Part model, mm, in its own coordinate system. A direction names the side the tool comes from. Round coordinates to 2 decimals unless told otherwise and drop trailing zeros. Loops run counter-clockwise (first coordinate to the right, second up) from the corner with the lowest first, then second, coordinate; pieces in that order, holes last. Notation, with made-up numbers: (-21, -9) - (-14, -9) arc R25 cw to (-14, 7) - close; hole circle Ø4 at (43, 51.25). An arc over 180 degrees is marked (long way). Write each question's results on one line, items separated by ' | '. Start each with the question number.
(1) Cut at A-A, the plane z = 8.75. List the corners of the cut face in (x, y), then the cut area to 3 significant figures.
(2) Tool access for faces 3 (the face through (-1.27, 0.97, 10.89)), 4 (the face through (-1.394, 2.37, 1.479)), 5 (the face through (-29.28, 9.514, 14.832)), 6 (the face through (-18.1, -24.91, 14.83)), 7 (the face through (-23.692, 20.716, 14.832)): list every direction of +Z, -Z, +X, -X, +Y, -Y with a clear straight run to the whole face (end or side of a thin tool).
(3) Flat gauge pins, fed straight in: P1, Ø4, axis at x = 0, y = 0, coming from the +Z side; P2, Ø3, axis at x = 0.5, y = -0.5, coming from the -Z side; P3, Ø6, axis at y = -13.5, z = 20.5, coming from the -X side. Where does each tip first touch, or does it go through?
(4) Drill centre lines: L1, parallel to Y at x = 14, z = 5.25; L2, parallel to Y at x = 11.5, z = 10.5; L3, parallel to Z at x = 8.5, y = -5.5. Where is each one in solid material? Low to high.
(5) Mould opens along Y. For faces 1 (the face through (-1.3, 1.4, 3)), 2 (the face through (-42.32, -28.46, 15.85)) say: released by +Y, released by -Y, zero draft, split by the parting line, or undercut.
from build123d import *

# Parameters (mm, degrees)
F0_R     = 51
F1_DEPTH = 3
F3_DEPTH = 24
F5_DEPTH = 3
F6_R     = 1.6
F7_DEPTH = 24.001
F8_R     = 7.5
F9_DEPTH = 8


# Not quite as in the source:
# - a fillet or chamfer that OpenCascade refuses, or shapes differently, is made with other operations: its cross-section is extruded or revolved along the edge and cut away or added


with BuildPart() as f1:
    # F0 (on Top) → F1 (new body)
    with BuildSketch(Plane.XY):
        Circle(F0_R)
    extrude(amount=F1_DEPTH)

    # F2 (on face) → F3 (join)
    with BuildSketch(Plane.XY.offset(3)):
        with BuildLine():
            Line((0, 51), (0, 10))
            ThreePointArc((0, 10), (0.6262291254, 9.9803725924), (1.25, 9.9215674165))
            ThreePointArc((1.25, 9.9215674165), (12.6111994349, 29.1522486886), (32.5125, 39.2929681209))
            ThreePointArc((32.5125, 39.2929681209), (17.2780008368, 47.9840670127), (0, 51))
        make_face()
        with BuildLine():
            Line((48.5038823311, 15.7598667131), (9.510565163, 3.0901699437))
            ThreePointArc((9.510565163, 3.0901699437), (9.6854138312, 2.4885254508), (9.8222425863, 1.8771122972))
            ThreePointArc((9.8222425863, 1.8771122972), (31.6225110248, -2.9854231318), (47.4167484056, -18.7790300773))
            ThreePointArc((47.4167484056, -18.7790300773), (50.0961783407, -9.5589181217), (51, 0))
            ThreePointArc((51, 0), (50.3721053704, 7.9781577171), (48.5038823311, 15.7598667131))
        make_face()
        with BuildLine():
            Line((29.9770478669, -41.2598667131), (5.8778525229, -8.0901699437))
            ThreePointArc((5.8778525229, -8.0901699437), (5.3596858173, -8.4423792819), (4.8204797641, -8.7614482161))
            ThreePointArc((4.8204797641, -8.7614482161), (6.9325871881, -30.9973416549), (-3.2073378494, -50.8990469844))
            ThreePointArc((-3.2073378494, -50.8990469844), (14.2261306293, -48.9756797535), (29.9770478669, -41.2598667131))
        make_face()
        with BuildLine():
            Line((-29.9770478669, -41.2598667131), (-5.8778525229, -8.0901699437))
            ThreePointArc((-5.8778525229, -8.0901699437), (-6.372945827, -7.7062027929), (-6.84302225, -7.2919850854))
            ThreePointArc((-6.84302225, -7.2919850854), (-27.3379365126, -16.1719875718), (-49.3989922099, -12.6783109541))
            ThreePointArc((-49.3989922099, -12.6783109541), (-42.1825232409, -28.6641715916), (-29.9770478669, -41.2598667131))
        make_face()
        with BuildLine():
            Line((-48.5038823311, 15.7598667131), (-9.510565163, 3.0901699437))
            ThreePointArc((-9.510565163, 3.0901699437), (-9.2983829469, 3.6796840317), (-9.0497001003, 4.2547535879))
            ThreePointArc((-9.0497001003, 4.2547535879), (-23.8283611351, 21.0025036698), (-27.3229183463, 43.0634198948))
            ThreePointArc((-27.3229183463, 43.0634198948), (-40.2963637234, 31.2602474506), (-48.5038823311, 15.7598667131))
        make_face()
        with BuildLine():
            ThreePointArc((-9.0497001003, 4.2547535879), (-4.6583345766, 1.8434602504), (0, 0))
            Line((0, 0), (0, 10))
            ThreePointArc((0, 10), (-5.3596858173, 8.4423792819), (-9.0497001003, 4.2547535879))
        make_face()
        with BuildLine():
            Line((-9.510565163, 3.0901699437), (0, 0))
            ThreePointArc((0, 0), (-4.6583345766, 1.8434602504), (-9.0497001003, 4.2547535879))
            ThreePointArc((-9.0497001003, 4.2547535879), (-9.2983829469, 3.6796840317), (-9.510565163, 3.0901699437))
        make_face()
        with BuildLine():
            ThreePointArc((-6.84302225, -7.2919850854), (-3.1927394333, -3.8606789083), (0, 0))
            Line((0, 0), (-9.510565163, 3.0901699437))
            ThreePointArc((-9.510565163, 3.0901699437), (-9.6854138312, -2.4885254508), (-6.84302225, -7.2919850854))
        make_face()
        with BuildLine():
            ThreePointArc((4.8204797641, -8.7614482161), (2.6851130896, -4.2294910354), (0, 0))
            Line((0, 0), (-5.8778525229, -8.0901699437))
            ThreePointArc((-5.8778525229, -8.0901699437), (-0.6262291254, -9.9803725924), (4.8204797641, -8.7614482161))
        make_face()
        with BuildLine():
            Line((-5.8778525229, -8.0901699437), (0, 0))
            ThreePointArc((0, 0), (-3.1927394333, -3.8606789083), (-6.84302225, -7.2919850854))
            ThreePointArc((-6.84302225, -7.2919850854), (-6.372945827, -7.7062027929), (-5.8778525229, -8.0901699437))
        make_face()
        with BuildLine():
            Line((5.8778525229, -8.0901699437), (0, 0))
            ThreePointArc((0, 0), (2.6851130896, -4.2294910354), (4.8204797641, -8.7614482161))
            ThreePointArc((4.8204797641, -8.7614482161), (5.3596858173, -8.4423792819), (5.8778525229, -8.0901699437))
        make_face()
        with BuildLine():
            ThreePointArc((9.8222425863, 1.8771122972), (4.8522305863, 1.2467096933), (0, 0))
            Line((0, 0), (5.8778525229, -8.0901699437))
            ThreePointArc((5.8778525229, -8.0901699437), (8.9100652419, -4.5399049974), (10, 0))
            ThreePointArc((10, 0), (9.9554614625, 0.9427550417), (9.8222425863, 1.8771122972))
        make_face()
        with BuildLine():
            Line((9.510565163, 3.0901699437), (0, 0))
            ThreePointArc((0, 0), (4.8522305863, 1.2467096933), (9.8222425863, 1.8771122972))
            ThreePointArc((9.8222425863, 1.8771122972), (9.6854138312, 2.4885254508), (9.510565163, 3.0901699437))
        make_face()
        with BuildLine():
            ThreePointArc((1.25, 9.9215674165), (0.313730334, 5), (0, 0))
            Line((0, 0), (9.510565163, 3.0901699437))
            ThreePointArc((9.510565163, 3.0901699437), (6.372945827, 7.7062027929), (1.25, 9.9215674165))
        make_face()
        with BuildLine():
            Line((0, 10), (0, 0))
            ThreePointArc((0, 0), (0.313730334, 5), (1.25, 9.9215674165))
            ThreePointArc((1.25, 9.9215674165), (0.6262291254, 9.9803725924), (0, 10))
        make_face()
    extrude(amount=F3_DEPTH)

    # F4 (on face) → F5 (cut)
    with BuildSketch(Plane(origin=(0, 0, 0), x_dir=(1, 0, 0), z_dir=(0, 0, -1))):
        Polygon((2.75, -1.5877132403), (2.75, 1.5877132403), (0, 3.1754264805), (-2.75, 1.5877132403), (-2.75, -1.5877132403), (0, -3.1754264805), align=None)
    extrude(amount=-F5_DEPTH, mode=Mode.SUBTRACT)

    # F6 (on face) → F7 (cut, through all)
    with BuildSketch(Plane(origin=(0, 0, 3), x_dir=(1, 0, 0), z_dir=(0, 0, -1))):
        Circle(F6_R)
    extrude(amount=-F7_DEPTH, mode=Mode.SUBTRACT)

    # F8 (on face) → F9 (cut)
    with BuildSketch(Plane.XY.offset(27)):
        Circle(F8_R)
    extrude(amount=-F9_DEPTH, mode=Mode.SUBTRACT)

    # F10: chamfer of 5 x 3.247037966 on 1 edges, made by hand

    # F10_s1 → F10_t2 (revolve, cut)
    with BuildSketch(Plane.XZ):
        Polygon((51, 5), (47.752962034, 0), (51, 0), align=None)
    revolve(axis=Axis((0, 0, 0), (0, 0, 1)), mode=Mode.SUBTRACT)


solid = f1.part
A:
1) outline: (-49.4, -12.68) arc R51 ccw to (-29.98, -41.26) - (-5.88, -8.09) arc R10 ccw to (4.82, -8.76) arc R40 cw to (-3.21, -50.9) arc R51 ccw to (29.98, -41.26) - (5.88, -8.09) arc R10 ccw to (9.82, 1.88) arc R40 cw to (47.42, -18.78) arc R51 ccw to (48.5, 15.76) - (9.51, 3.09) arc R10 ccw to (1.25, 9.92) arc R40 cw to (32.51, 39.29) arc R51 ccw to (0, 51) - (0, 10) arc R10 ccw to (-9.05, 4.25) arc R40 cw to (-27.32, 43.06) arc R51 ccw to (-48.5, 15.76) - (-9.51, 3.09) arc R10 ccw to (-6.84, -7.29) arc R40 cw to start; hole circle Ø3.2 at (0, 0) | area: 3,180 mm2
2) face 3: +Z, -Z | face 4: -Z | face 5: +Z, -X | face 6: +Z, -Y | face 7: +Z
3) P1: z = 19 | P2: z = 3 | P3: x = -49.4
4) L1: -49.04 to -19.27, 1.92 to 4.55, 30.4 to 49.04 | L2: -49.69 to -15.83, 1.95 to 3.74, 28.07 to 49.69 | L3: 0 to 3
5) face 1: undercut | face 2: released by -Y
